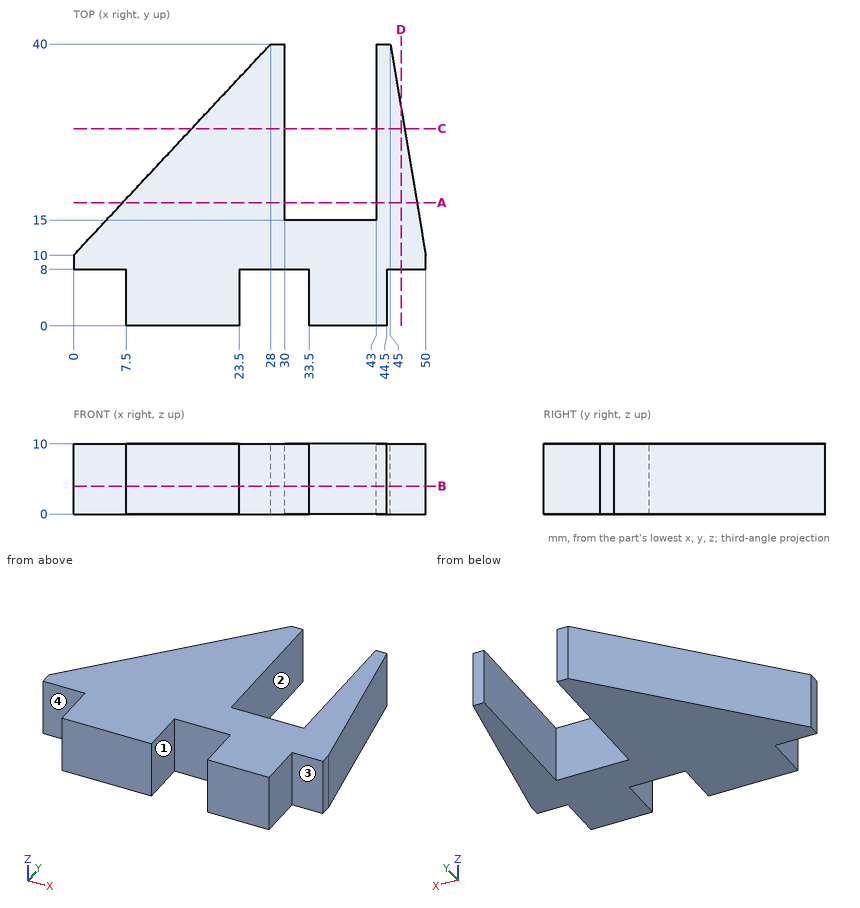
Answer from the drawing. Dimensions are ordinates in mm from the lowest x, y and z of the part. A direction names the side the tool comes from. Coordinates: 2 decimals unless noted, no trailing zeros. Write each loop counter-clockwise with the first axis right and the second up, starting at its lowest first coordinate (ties: lowest second). Pieces come first, ordered by that corner, then holes. Notation, with made-up numbers: M 4.25,52.5 L 18.25,52.5 A21 cw 18.25,82.5 Z; hole C 3.25,-20.75 d4. An arc over 180 degrees is marked long. Use one line per item in the form item = value. Start each with the question number.
1. The part is cut by section C-C (y = 28). Give the vertices of the cut face in (x, z), plus the area to 3 significant figures.
2. Each of these flat-tipped pins is pushed along its axis until it touches: P1, Ø2.5, axis at y = 3.5, z = 6.5, coming from the +X side; P2, Ø4, axis at y = 5.5, z = 7, coming from the -X side; P3, Ø1, axis at x = 26.5, z = 6.5, coming from the -Y side. Where does it stop, or does it pass through?
3. The part is cut by section B-B (z = 4). Give the vertices of the cut face in (x, y), plus the area to 3 significant figures.
4. A tool of negligible diameter and unlimited length cuts with its end or side. For the marked faces 1, 2, 3 and 4, from which of +Z, -Z, +X, -X, +Y, -Y can it reach the whole face along a straight path? Write none if from no direction.
5. The part is cut by section A-A (y = 17.5). Give the vertices of the cut face in (x, z), plus the area to 4 significant figures.
6. Straight lines are drawn through the part: probe 1 along X at (y, z) = (3.5, 3); probe 2 along Y at (x, z) = (37, 3.5); probe 3 along X at (y, z) = (16, 4). For each, find the intervals that lie inside material, in ascending order. Write a range as from..to.
7. The part is cut by section D-D (x = 46.5). Give the vertices of the cut face in (y, z), plus the area to 3 significant figures.
Evaluation:
q1.outline = M 16.8,0 L 30,0 L 30,10 L 16.8,10 Z; M 43,0 L 47,0 L 47,10 L 43,10 Z
q1.area = 172 mm^2
q2.P1 = 44.5
q2.P2 = 7.5
q2.P3 = 8
q3.outline = M 0,8 L 7.5,8 L 7.5,0 L 23.5,0 L 23.5,8 L 33.5,8 L 33.5,0 L 44.5,0 L 44.5,8 L 50,8 L 50,10 L 45,40 L 43,40 L 43,15 L 30,15 L 30,40 L 28,40 L 0,10 Z
q3.area = 996 mm^2
q4.face_1 = +Z, -Z, -Y
q4.face_2 = +Z, -Z, +Y
q4.face_3 = +Z, -Z, +X, -Y
q4.face_4 = +Z, -Z, -X, -Y
q5.outline = M 7,0 L 30,0 L 30,10 L 7,10 Z; M 43,0 L 48.75,0 L 48.75,10 L 43,10 Z
q5.area = 287.5 mm^2
q6.probe_1 = 7.5..23.5, 33.5..44.5
q6.probe_2 = 0..15
q6.probe_3 = 5.6..30, 43..49
q7.outline = M 8,0 L 31,0 L 31,10 L 8,10 Z
q7.area = 230 mm^2
